from build123d import *

# Parameters (mm, degrees)
EXTRUDE_1_DEPTH     = 20
SKETCH_2_W          = 13
SKETCH_2_H          = 3
EXTRUDE_2_DEPTH     = 20
SKETCH_5_W          = 3
SKETCH_5_H          = 40
EXTRUDE_3_DEPTH     = 60
CUT_EXTRUDE_1_REACH = 113.283
SKETCH_6_R          = 4
SKETCH_6_R_2        = 1.75


# Read off the part's stored shape, not the designer's step: M3 すきま穴1
with BuildPart() as part:
    # ｽｹｯﾁ1 → ﾎﾞｽ - 押し出し1 (new body)
    with BuildSketch(Plane.XY):
        with BuildLine():
            Line((-23, 0), (-26, 0))
            ThreePointArc((-26, 0), (0, 26), (26, 0))
            Line((26, 0), (23, 0))
            ThreePointArc((23, 0), (0, 23), (-23, 0))
        make_face()
    extrude(amount=EXTRUDE_1_DEPTH)

    # ｽｹｯﾁ2 → ﾎﾞｽ - 押し出し2 (add)
    with BuildSketch(Plane.XY.offset(20)):
        with Locations((-29.5, 1.5)):
            Rectangle(SKETCH_2_W, SKETCH_2_H)
        with Locations((29.5, 1.5)):
            Rectangle(SKETCH_2_W, SKETCH_2_H)
    extrude(amount=-EXTRUDE_2_DEPTH)

    # M3 すきま穴1 outline → M3 すきま穴1 (revolve, cut)
    with BuildSketch(Plane(origin=(31, 0, 15), x_dir=(1, 0, 0), z_dir=(0, 0, 1))):
        Polygon((0, 0), (1.7, 0), (1.7, 2.97124079), (1.725, 3), (0, 3), align=None)
    revolve(axis=Axis((31, 0, 15), (0, 1, 0)), mode=Mode.SUBTRACT)

    # Hole Wizard M3 _1 2 outline → Hole Wizard M3 _1 2 (revolve, cut)
    with BuildSketch(Plane(origin=(31, 0, 5), x_dir=(1, 0, 0), z_dir=(0, 0, 1))):
        Polygon((0, 0), (1.7, 0), (1.7, 2.97124079), (1.725, 3), (0, 3), align=None)
    revolve(axis=Axis((31, 0, 5), (0, 1, 0)), mode=Mode.SUBTRACT)

    # Hole Wizard M3 _1 3 outline → Hole Wizard M3 _1 3 (revolve, cut)
    with BuildSketch(Plane(origin=(-31, 0, 15), x_dir=(1, 0, 0), z_dir=(0, 0, 1))):
        Polygon((0, 0), (1.7, 0), (1.7, 2.97124079), (1.725, 3), (0, 3), align=None)
    revolve(axis=Axis((-31, 0, 15), (0, 1, 0)), mode=Mode.SUBTRACT)

    # Hole Wizard M3 _1 4 outline → Hole Wizard M3 _1 4 (revolve, cut)
    with BuildSketch(Plane(origin=(-31, 0, 5), x_dir=(1, 0, 0), z_dir=(0, 0, 1))):
        Polygon((0, 0), (1.7, 0), (1.7, 2.97124079), (1.725, 3), (0, 3), align=None)
    revolve(axis=Axis((-31, 0, 5), (0, 1, 0)), mode=Mode.SUBTRACT)

    # ｽｹｯﾁ5 → ﾎﾞｽ - 押し出し3 (add)
    with BuildSketch(Plane.XZ):
        with Locations((34.5, 40)):
            Rectangle(SKETCH_5_W, SKETCH_5_H)
    extrude(amount=-EXTRUDE_3_DEPTH)

    # ｽｹｯﾁ6 → ｶｯﾄ - 押し出し1 (cut, up to next)
    with BuildSketch(Plane(origin=(36, 0, 0), x_dir=(0, 0, -1), z_dir=(1, 0, 0)), mode=Mode.PRIVATE) as cut_extrude_1_sk1:
        with Locations((-40, 40)):
            Circle(SKETCH_6_R)
    cut_extrude_1_tool1 = extrude(cut_extrude_1_sk1.sketch, amount=-CUT_EXTRUDE_1_REACH, mode=Mode.PRIVATE) & part.part
    # ｽｹｯﾁ6 → ｶｯﾄ - 押し出し1 (cut, up to next)
    with BuildSketch(Plane(origin=(36, 0, 0), x_dir=(0, 0, -1), z_dir=(1, 0, 0)), mode=Mode.PRIVATE) as cut_extrude_1_sk2:
        with Locations((-24.5, 55.5)):
            Circle(SKETCH_6_R_2)
    cut_extrude_1_tool2 = extrude(cut_extrude_1_sk2.sketch, amount=-CUT_EXTRUDE_1_REACH, mode=Mode.PRIVATE) & part.part
    # ｽｹｯﾁ6 → ｶｯﾄ - 押し出し1 (cut, up to next)
    with BuildSketch(Plane(origin=(36, 0, 0), x_dir=(0, 0, -1), z_dir=(1, 0, 0)), mode=Mode.PRIVATE) as cut_extrude_1_sk3:
        with Locations((-24.5, 24.5)):
            Circle(SKETCH_6_R_2)
    cut_extrude_1_tool3 = extrude(cut_extrude_1_sk3.sketch, amount=-CUT_EXTRUDE_1_REACH, mode=Mode.PRIVATE) & part.part
    # ｽｹｯﾁ6 → ｶｯﾄ - 押し出し1 (cut, up to next)
    with BuildSketch(Plane(origin=(36, 0, 0), x_dir=(0, 0, -1), z_dir=(1, 0, 0)), mode=Mode.PRIVATE) as cut_extrude_1_sk4:
        with Locations((-55.5, 24.5)):
            Circle(SKETCH_6_R_2)
    cut_extrude_1_tool4 = extrude(cut_extrude_1_sk4.sketch, amount=-CUT_EXTRUDE_1_REACH, mode=Mode.PRIVATE) & part.part
    # ｽｹｯﾁ6 → ｶｯﾄ - 押し出し1 (cut, up to next)
    with BuildSketch(Plane(origin=(36, 0, 0), x_dir=(0, 0, -1), z_dir=(1, 0, 0)), mode=Mode.PRIVATE) as cut_extrude_1_sk5:
        with Locations((-55.5, 55.5)):
            Circle(SKETCH_6_R_2)
    cut_extrude_1_tool5 = extrude(cut_extrude_1_sk5.sketch, amount=-CUT_EXTRUDE_1_REACH, mode=Mode.PRIVATE) & part.part
    add(cut_extrude_1_tool1.solids().sort_by_distance((36, 40, 40))[0], mode=Mode.SUBTRACT)
    add(cut_extrude_1_tool2.solids().sort_by_distance((36, 55.5, 24.5))[0], mode=Mode.SUBTRACT)
    add(cut_extrude_1_tool3.solids().sort_by_distance((36, 24.5, 24.5))[0], mode=Mode.SUBTRACT)
    add(cut_extrude_1_tool4.solids().sort_by_distance((36, 24.5, 55.5))[0], mode=Mode.SUBTRACT)
    add(cut_extrude_1_tool5.solids().sort_by_distance((36, 55.5, 55.5))[0], mode=Mode.SUBTRACT)


solid = part.part
Design review of the part built by this model. Coordinates are the model's own, in mm. A direction names the side the tool comes from. Coordinates: 2 decimals unless noted, no trailing zeros. Loops run counter-clockwise (first coordinate to the right, second up) from the corner with the lowest first, then second, coordinate; pieces in that order, holes last. Notation, with made-up numbers: M 39,2.5 L 90,2.5 A12 cw 90,6.5 Z; hole C 43.25,-13.5 d11. An arc over 180 degrees is marked long. Use one line per item in the form item = value.
(1) Consider section D-D (y = 40). Write out the cut boundary in (x, z).
Return value:
outline = M 33,20 L 36,20 L 36,36 L 33,36 Z; M 33,44 L 36,44 L 36,60 L 33,60 Z
(2) Consider section A-A (z = 24.5). Write out the cut boundary in (x, y), and give its area (3 significant figures).
Return value:
outline = M 33,0 L 36,0 L 36,22.75 L 33,22.75 Z; M 33,26.25 L 36,26.25 L 36,53.75 L 33,53.75 Z; M 33,57.25 L 36,57.25 L 36,60 L 33,60 Z
area = 159 mm2
(3) Consider section B-B (y = 55.5). Write out the cut boundary in (x, z).
Return value:
outline = M 33,20 L 36,20 L 36,22.75 L 33,22.75 Z; M 33,26.25 L 36,26.25 L 36,53.75 L 33,53.75 Z; M 33,57.25 L 36,57.25 L 36,60 L 33,60 Z
(4) Draft analysis for pull direction X (two halves, no side actions). For faces 4 (the face through (-29.38, 1.51, 14.49)), 5 (the face through (33, 30, 40)), 6 (the face through (-0.53, 25.995, 9.86)), 7 (the face through (34, 60, 40)), state which applies: pulls with the +X half, pulls with the -X half, needs draft (parallel to the pull), parting line crosses it, or undercut.
Return value:
face_4 = undercut
face_5 = pulls with the -X half
face_6 = parting line crosses it
face_7 = needs draft
(5) Clearance check with flat-ended pins moving along their axes: P1, Ø2, axis at x = -31, z = 15, coming from the -Y side; P2, Ø10, axis at x = 14, y = 18, coming from the -Z side; P3, Ø8, axis at x = -15.5, y = 14, coming from the +Z side; P4, Ø5.5, axis at x = -31, z = 5, coming from the +Y side. State where each tip first meets the part, or that it passes through.
Return value:
P1 = through
P2 = 0
P3 = 20
P4 = 3
(6) Consider section C-C (x = 31). Write out the cut boundary in (y, z) (3 decimals), and give its area (3 significant figures).
Return value:
outline = M 0,0 L 3,0 L 3,3.275 L 2.971,3.3 L 0,3.3 Z; M 0,6.7 L 2.971,6.7 L 3,6.725 L 3,13.275 L 2.971,13.3 L 0,13.3 Z; M 0,16.7 L 2.971,16.7 L 3,16.725 L 3,20 L 0,20 Z
area = 39.6 mm2
(7) For line 1 along Y through (x, z) = (35.25, 24.5); line 2 along Z through (x, y) = (33.5, 57.5); line 3 along X through (y, z) = (31, 22), list the stretches that pass through material, from the lowest coordinate up. Write a range as from..to.
Return value:
line_1 = 0..22.75, 26.25..53.75, 57.25..60
line_2 = 20..60
line_3 = 33..36
(8) For faces 1 (the face through (-2, 24, 20)), 2 (the face through (31, 3, 10)), 3 (the face through (31, 0, 17)), list the 3-axis set-ups (+Z, -Z, +X, -X, +Y, -Y) from which the entire face can be reached by the end or side of a thin tool; tool diameter is ignored.
Return value:
face_1 = +Z, -X, +Y, -Y
face_2 = -Z, +X, +Y
face_3 = +Z, -Z, +X, -X, -Y
